The model under review builds one solid part; all positions refer to its coordinate system, in mm. Face numbers are marked on the shaded views. A direction names the side the tool comes from. Give positions to 0.01 mm unless a question says otherwise; leave off trailing zeros. Order: outer loops, then holes, each group sorted by start corner. A loop starts at its lowest first (then second) coordinate and runs counter-clockwise, first axis right, second up. Notation, with made-up numbers: M -28.75,-27 L -18.75,-27 A28 cw -18.75,11 Z; hole C -34.5,-9 d1. An arc over 180 degrees is marked long. One line per question, with ' | ' between items. Start each with the question number.
1. The part is to be moulded in two halves that separate along Z. For the marked faces 1 and 2, say which applies: +Z half, -Z half, draft (parallel to the pull), parting line (faces both ways), or undercut.
2. We need section B-B on x = 0. Write out the cut boundary in (y, z), then the cut area to 3 significant figures.
3. Insertion check: P1, Ø3, axis at x = 8.5, z = -6.5, coming from the -Y side; P2, Ø2, axis at x = -15, z = 11.5, coming from the +Y side; P3, Ø3, axis at y = -1, z = -4.5, coming from the -X side; P4, Ø1.5, axis at y = -2.5, z = -3, coming from the +X side. Each pin has a flat end and moves straight along its axis. Give the tip position at first contact, or say it passes through.
4. For the marked faces 3 and 4, list the 3-axis set-ups (+Z, -Z, +X, -X, +Y, -Y) from which the entire face can be reached by the end or side of a thin tool; tool diameter is ignored.
5. Wall thickness on L1, parallel to X at y = -4.6, z = -4.5; L2, parallel to X at y = -0.35, z = 1.5; L3, parallel to Z at x = -3, y = -3.95: over which ranges is each line inside the solid? List them lowest first.
6. We need section C-C on z = 10. Count the separate pieces of the cut face and the enclosed holes in it, then the cut area to 3 significant figures.
7. We need section A-A on z = 0. Write out the cut boundary in (x, y).
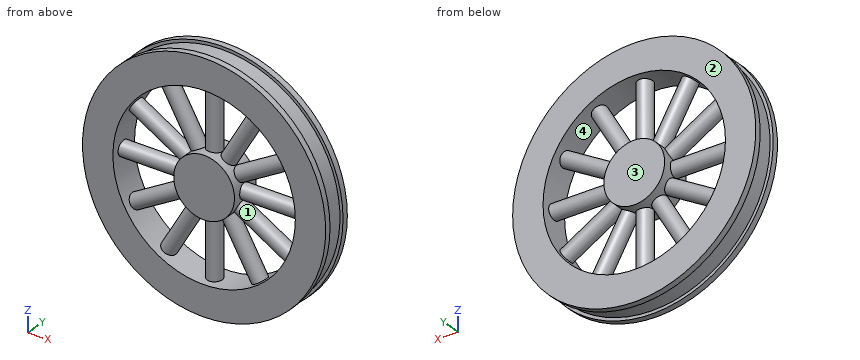
```python
from build123d import *

# Parameters (mm, degrees)
F0_R            = 20
F1_DEPTH        = 5
F2_R            = 15
F3_DEPTH        = 5
F4_R            = 5
F5_DEPTH        = 5
F6_R            = 1.25
F7_DEPTH        = 19
F7_COPIES_COUNT = 12
F8_W            = 3
F8_H            = 0.5


# Not quite as in the source:
# - a pattern or mirror of a feature is missing from the dataset's text; its kind, count and spacing are read off the source's solid


with BuildPart() as f1:
    # F0 (on Front) → F1 (new body)
    with BuildSketch(Plane.XZ):
        Circle(F0_R)
    extrude(amount=F1_DEPTH)

    # F2 (on face) → F3 (cut)
    with BuildSketch(Plane.XZ.offset(5)):
        Circle(F2_R)
    extrude(amount=-F3_DEPTH, mode=Mode.SUBTRACT)



with BuildPart() as f5:
    # F4 (on Front) → F5 (new body)
    with BuildSketch(Plane.XZ):
        Circle(F4_R)
    extrude(amount=F5_DEPTH)


with BuildPart() as f1_1:
    add(f1.part)

    add(f5.part)  # F7 merges F5
    # F6 (on Right) → F7 (join)
    with BuildSketch(Plane.YZ):
        with Locations((-2.5505366686, 0)):
            Circle(F6_R)
    f7 = extrude(amount=F7_DEPTH)

    # F7_copies: F7 ×12 about axis
    f7_copies_axis = Axis((0, 0, 0), (0, 1, 0))
    for i in range(1, F7_COPIES_COUNT):
        add(f7.rotate(f7_copies_axis, i * 360 / F7_COPIES_COUNT))

    # F8 (on Right) → F9 (revolve, cut)
    with BuildSketch(Plane.YZ):
        with Locations((-2.5, 19.75)):
            Rectangle(F8_W, F8_H)
    revolve(axis=Axis((0, 0, 0), (0, 1, 0)), mode=Mode.SUBTRACT)


solid = f1_1.part
```
Entries:
1) face 1: undercut | face 2: draft
2) outline: M -5,-20 L -4,-20 L -4,-19.5 L -1,-19.5 L -1,-20 L 0,-20 L 0,-15 L -1.3,-15 L -1.3,-5 L 0,-5 L 0,5 L -1.3,5 L -1.3,15 L 0,15 L 0,20 L -1,20 L -1,19.5 L -4,19.5 L -4,20 L -5,20 L -5,15 L -3.8,15 L -3.8,5 L -5,5 L -5,-5 L -3.8,-5 L -3.8,-15 L -5,-15 Z | area: 147 mm^2
3) P1: stops at y = -3.8 | P2: stops at y = 0 | P3: stops at x = -19.77 | P4: stops at x = 19.37
4) face 3: +Z, -Z, +X, -X, +Y | face 4: none
5) L1: x = -19.49 to -14.31, -2.18 to 2.18, 14.31 to 19.49 | L2: x = -19.94 to -14.92, -4.77 to 4.77, 14.92 to 19.94 | L3: z = -19.27 to -14.7, -4 to 4, 14.7 to 19.27
6) separate pieces: 5 | enclosed holes: 0 | area: 74.2 mm^2
7) outline: M -20,-5 L -15,-5 L -15,-3.8 L -5,-3.8 L -5,-5 L 5,-5 L 5,-3.8 L 15,-3.8 L 15,-5 L 20,-5 L 20,-4 L 19.5,-4 L 19.5,-1 L 20,-1 L 20,0 L 15,0 L 15,-1.3 L 5,-1.3 L 5,0 L -5,0 L -5,-1.3 L -15,-1.3 L -15,0 L -20,0 L -20,-1 L -19.5,-1 L -19.5,-4 L -20,-4 Z
